Autodesk Inventor part; units mm, degrees
ref_plane "YZ Plane" through (0, 0, 0) normal (1, 0, 0) x (0, 1, 0)
ref_plane "XZ Plane" through (0, 0, 0) normal (0, 1, 0) x (-1, 0, 0)
ref_plane "XY Plane" through (0, 0, 0) normal (0, 0, 1) x (1, 0, 0)
sketch "Sketch1" plane through (0, 0, 0) normal (0, 1, 0) x (-1, 0, 0)
  line L0 (0, 0) -> (-190, 0)
  line L1 (-190, 0) -> (-190, -40)
  line L2 (-190, -40) -> (0, -40)
  line L3 (0, -40) -> (0, 0)
  dimension "d0" = 190
  dimension "d1" = 40
extrude "Extrusion1" add sketch "Sketch1" along normal blind 5
sketch "Sketch2" plane through (0, 5, 0) normal (0, 1, 0) x (1, 0, 0)
  line L0 (20, 17.5) -> (0, 17.5)
  line L1 (0, 17.5) -> (0, 22.5)
  line L2 (0, 22.5) -> (20, 22.5)
  line L3 (20, 22.5) -> (20, 17.5)
  line L4 (170, 22.5) -> (190, 22.5)
  line L5 (190, 22.5) -> (190, 17.5)
  line L6 (190, 17.5) -> (170, 17.5)
  line L7 (170, 17.5) -> (170, 22.5)
  line L8 (0, 40) -> (0, 0)
  line L9 (190, 0) -> (190, 40)
  point P0 (0, 20)
  point P1 (0, 20)
  point P2 (190, 20)
  point P3 (190, 20)
  point P4 (0, 20)
  point P5 (190, 20)
  dimension "d4" = 20
  dimension "d5" = 5
  dimension "d6" = 20
  dimension "d7" = 5
extrude "Extrusion2" add sketch "Sketch2" along normal blind 90
sketch "Sketch3" plane through (0, 5, 0) normal (0, 1, 0) x (1, 0, 0)
  circle A0 centre (65, 20) radius 4
  circle A1 centre (125, 20) radius 4
  line L0 (0, 22.5) -> (0, 17.5)
  line L1 (65, 20) -> (125, 20) construction
  line L2 (0, 0) -> (190, 0)
  point P0 (0, 20)
  point P1 (95, 20)
  point P2 (95, 0)
  dimension "d10" = 8
  dimension "d11" = 8
  dimension "d12" = 60
extrude "Extrusion3" cut sketch "Sketch3" against normal blind 90
sketch "Sketch4" plane through (170, 5, -17.5) normal (0, 0, 1) x (1, 0, 0)
  circle A0 centre (10, 20) radius 2.5
  circle A1 centre (10, 70) radius 2.5
  circle A2 centre (-160, 70) radius 2.5
  circle A3 centre (-160, 20) radius 2.5
  line L0 (0, 90) -> (20, 90)
  line L1 (-170, 90) -> (-150, 90)
  point P0 (-170, -5)
  point P1 (10, 90)
  point P2 (-160, 90)
  dimension "d17" = 5
  dimension "d18" = 5
  dimension "d19" = 5
  dimension "d20" = 5
  dimension "d21" = 50
  dimension "d22" = 50
  dimension "d23" = 20
  dimension "d24" = 20
extrude "Extrusion4" cut sketch "Sketch4" against normal blind 90
equation "\"d22\" = d21"
properties part number "X-Axis Panel Mount" material "Steel"
Here's how the part is built. I have some questions about the finished solid (model axes, mm). A direction names the side the tool comes from. Coordinates: 2 decimals unless noted, no trailing zeros. Loops run counter-clockwise (first coordinate to the right, second up) from the corner with the lowest first, then second, coordinate; pieces in that order, holes last. Notation, with made-up numbers: (-29.75, -1.5) -> (19.25, -1.5) arc R10 cw to (19.25, 17.5) -> close; hole circle Ø8 at (-22, -21). An arc over 180 degrees is marked (long way). Use one line per item in the form item = value. Start each with the question number.
(1) If we section it at B-B (y = 41): Please give me the cut outline in (x, z).
(2) If we section it at D-D (y = 25): Please give me the cut outline in (x, z).
(3) If we section it at A-A (z = -20): Please give me the cut outline in (x, y).
(4) Will these pins go through, and if not, where does the flat tip stop? pin 1 (8 mm diameter, centred on x = 10, y = 25, fed in from +Z); pin 2 (5 mm diameter, centred on x = 131, z = -17.5, fed in from +Y); pin 3 (3 mm diameter, centred on x = 10, y = 75, fed in from +Z); pin 4 (22 mm diameter, centred on x = 11, y = 39.5, fed in from -Z).
(5) Please list where these lines run through material, in increasing order: line 1 along Y through (x, z) = (180, -20.15); line 2 along X through (y, z) = (1.55, -20); line 3 along X through (y, z) = (62, -20).
(6) If we section it at C-C (x = 10): Please give me the cut outline in (y, z), then the cut area to 3 significant figures.
(7) On a 3-axis mill with a long thin cutter (end or side, diameter ignored), from which of +Z, -Z, +X, -X, +Y, -Y can I reach the whole of each face in a straight line? I mean faces 1 (the face through (10, 49, -17.5)), 2 (the face through (180, 49, -22.5)), 3 (the face through (20, 49, -20)). Say none if no direction works.
(8) We'd pull the mould along Z, two halves only. Please class faces 4 (the face through (68.815, 2.535, -21.201)), 5 (the face through (180, 49, -17.5)), 6 (the face through (180, 95, -20)): pulls with the +Z half, pulls with the -Z half, needs draft (parallel to the pull), parting line crosses it, or undercut.
Verdict:
q1.outline = (0, -22.5) -> (20, -22.5) -> (20, -17.5) -> (0, -17.5) -> close; (170, -22.5) -> (190, -22.5) -> (190, -17.5) -> (170, -17.5) -> close
q2.outline = (0, -22.5) -> (7.5, -22.5) -> (7.5, -17.5) -> (0, -17.5) -> close; (12.5, -22.5) -> (20, -22.5) -> (20, -17.5) -> (12.5, -17.5) -> close; (170, -22.5) -> (177.5, -22.5) -> (177.5, -17.5) -> (170, -17.5) -> close; (182.5, -22.5) -> (190, -22.5) -> (190, -17.5) -> (182.5, -17.5) -> close
q3.outline = (0, 0) -> (61, 0) -> (61, 5) -> (20, 5) -> (20, 95) -> (0, 95) -> close; (69, 0) -> (121, 0) -> (121, 5) -> (69, 5) -> close; (129, 0) -> (190, 0) -> (190, 95) -> (170, 95) -> (170, 5) -> (129, 5) -> close; hole circle Ø5 at (10, 25); hole circle Ø5 at (10, 75); hole circle Ø5 at (180, 25); hole circle Ø5 at (180, 75)
q4.pin_1 = -17.5
q4.pin_2 = 5
q4.pin_3 = through
q4.pin_4 = -22.5
q5.line_1 = 0 to 22.5, 27.5 to 72.5, 77.5 to 95
q5.line_2 = 0 to 61, 69 to 121, 129 to 190
q5.line_3 = 0 to 20, 170 to 190
q6.outline = (0, -40) -> (5, -40) -> (5, -22.5) -> (22.5, -22.5) -> (22.5, -17.5) -> (5, -17.5) -> (5, 0) -> (0, 0) -> close; (27.5, -22.5) -> (72.5, -22.5) -> (72.5, -17.5) -> (27.5, -17.5) -> close; (77.5, -22.5) -> (95, -22.5) -> (95, -17.5) -> (77.5, -17.5) -> close
q6.area = 600 mm²
q7.face_1 = +Z, +X, -X, +Y
q7.face_2 = -Z, +X, -X, +Y
q7.face_3 = +Z, -Z, +Y
q8.face_4 = undercut
q8.face_5 = pulls with the +Z half
q8.face_6 = needs draft
